from build123d import *

# Parameters (mm, degrees)
F0_R      = 12.7
F1_DEPTH  = 30.1625
F2_W      = 56.912827603
F2_H      = 22.3266
F3_DEPTH  = 44.705
F4_R      = 3.302
F5_R      = 3.302
F6_R      = 6.35
F7_DEPTH  = 22.353
F9_DEPTH  = 19.05
F11_DEPTH = 19.05
F12_R     = 7.874
F13_R     = 5.08


with BuildPart() as f1:
    # F0 (on Front) → F1 (new body, symmetric)
    with BuildSketch(Plane.XZ):
        with BuildLine():
            ThreePointArc((22.352, 22.352), (-15.8052507731, 38.1572507731), (0, 0))
            Line((0, 0), (194.2084, 0))
            Line((194.2084, 0), (194.2084, 22.352))
            Line((194.2084, 22.352), (22.352, 22.352))
        make_face()
        with Locations((0, 22.352)):
            Circle(F0_R, mode=Mode.SUBTRACT)
    extrude(amount=F1_DEPTH, both=True)

    # F2 (on Top) → F3 (cut, through all)
    with BuildSketch(Plane.XY):
        Rectangle(F2_W, F2_H)
    extrude(amount=F3_DEPTH, mode=Mode.SUBTRACT)

    # F4
    f4_edges = [f1.edges().sort_by_distance(p)[0] for p in [
        (22.352, 20.6629, 22.352),
    ]]
    fillet(f4_edges, radius=F4_R)

    # F5
    f5_edges = [f1.edges().sort_by_distance(p)[0] for p in [
        (22.352, -20.6629, 22.352),
    ]]
    fillet(f5_edges, radius=F5_R)

    # F6 (on face) → F7 (cut, through all)
    with BuildSketch(Plane.XY.offset(22.352)):
        with Locations((155.3464, 15.4305)):
            Circle(F6_R)
    extrude(amount=-F7_DEPTH, mode=Mode.SUBTRACT)

    # F8 (on face) → F9 (cut)
    with BuildSketch(Plane.XZ.offset(30.1625)):
        Polygon((117.2464, 0), (117.2464, 22.352), (85.852, 22.352), (91.8464, 0), align=None)
    extrude(amount=-F9_DEPTH, mode=Mode.SUBTRACT)

    # F10 (on face) → F11 (join)
    with BuildSketch(Plane.XZ.offset(30.1625)):
        with BuildLine():
            ThreePointArc((130.1968694519, 57.15), (127.0147572456, 38.5254271914), (117.2464, 22.352))
            Line((117.2464, 22.352), (150.0886, 22.352))
            Line((150.0886, 22.352), (153.3906, 22.352))
            ThreePointArc((153.3906, 22.352), (151.0557334085, 23.3191334085), (150.0886, 25.654))
            Line((150.0886, 25.654), (150.0886, 57.15))
            Line((150.0886, 57.15), (130.1968694519, 57.15))
        make_face()
    extrude(amount=-F11_DEPTH)

    # F12
    f12_edges = [f1.edges().sort_by_distance(p)[0] for p in [
        (194.2084, 0, 22.352),
    ]]
    fillet(f12_edges, radius=F12_R)

    # F13
    f13_edges = [f1.edges().sort_by_distance(p)[0] for p in [
        (150.0886, -20.6375, 57.15),
    ]]
    fillet(f13_edges, radius=F13_R)


solid = f1.part
CAD build for the part. Positions are in the model's coordinates, mm. A direction names the side the tool comes from. Give positions to 0.01 mm unless a question says otherwise; leave off trailing zeros. Loops run counter-clockwise (first coordinate to the right, second up) from the corner with the lowest first, then second, coordinate; pieces in that order, holes last. Notation, with made-up numbers: M 29,15.5 L 47,15.5 A6 ccw 47,25.5 Z; hole C 80,23 d3. An arc over 180 degrees is marked long. Write each question's results on one line, items separated by ' | '.
Q1. Flat gauge pins, fed straight in: P1, Ø4, axis at x = 89, z = 19, coming from the -Y side; P2, Ø15, axis at y = -22, z = 38, coming from the +X side; P3, Ø15, axis at x = 0, z = 22.352, coming from the +Y side; P4, Ø5.5, axis at y = -21.5, z = 9.5, coming from the -X side. Where does each tip first touch, or does it go through?
Geometry check:
P1: stops at y = -11.11 | P2: stops at x = 150.09 | P3: passes through | P4: stops at x = -19.94
Q2. Band-saw the part on D-D on x = 101. Write the cut outline in (y, z), and give its area (3 significant figures).
Geometry check:
outline: M -11.11,0 L 30.16,0 L 30.16,22.35 L -11.11,22.35 Z | area: 923 mm²
Q3. Band-saw the part on B-B on x = -6. Write the cut outline in (y, z), and give its area (3 significant figures).
Geometry check:
outline: M -30.16,0.82 L -11.16,0.82 L -11.16,11.16 L -30.16,11.16 Z; M -30.16,33.55 L -11.16,33.55 L -11.16,43.88 L -30.16,43.88 Z; M 11.16,0.82 L 30.16,0.82 L 30.16,11.16 L 11.16,11.16 Z; M 11.16,33.55 L 30.16,33.55 L 30.16,43.88 L 11.16,43.88 Z | area: 786 mm²
Q4. Band-saw the part on C-C on y = 0. Write the cut outline in (x, z), and give its area (3 significant figures).
Geometry check:
outline: M 28.46,0 L 194.21,0 L 194.21,14.48 A7.87 ccw 186.33,22.35 L 28.46,22.35 Z | area: 3,690 mm²
Q5. Which spindle directions (+Z, -Z, +X, -X, +Y, -Y) get a long thin tool onto all of the face, cutting with end or side? Do faces 5 (the face through (107, 0, 22.352)), 6 (the face through (88.807, -20.771, 11.332)), 7 (the face through (150.089, -21, 39)), 8 (the face through (139, -11.112, 40)). Say none if no direction does.
Geometry check:
face 5: +Z, +Y | face 6: +Z, -Y | face 7: +Z, +X, +Y, -Y | face 8: +Z, +X, -X, +Y
Q6. Band-saw the part on A-A on z = 28.5. Write the cut outline in (x, y).
Geometry check:
outline: M -21.49,-30.16 L -11.11,-30.16 L -11.11,-11.16 L -21.49,-11.16 Z; M -21.49,11.16 L -11.11,11.16 L -11.11,30.16 L -21.49,30.16 Z; M 11.11,-30.16 L 21.49,-30.16 L 21.49,-11.16 L 11.11,-11.16 Z; M 11.11,11.16 L 21.49,11.16 L 21.49,30.16 L 11.11,30.16 Z; M 121.96,-30.16 L 150.09,-30.16 L 150.09,-11.11 L 121.96,-11.11 Z
Q7. Mould opens along X. For faces 1 (the face through (127.11, -20.77, 38.78)), 2 (the face through (148.64, -20.5, 55.62)), 3 (the face through (-16.31, 20.53, 37.636)), 4 (the face through (34, -30.162, 18)) say: pulls with the +X half, pulls with the -X half, needs draft (parallel to the pull), parting line crosses it, or undercut.
Geometry check:
face 1: undercut | face 2: pulls with the +X half | face 3: parting line crosses it | face 4: needs draft
Q8. Probe probe 1 along Y at (x, z) = (28, 20); probe 2 along Z at (x, y) = (0, 24.5); probe 3 along X at (y, z) = (-13.5, 31). List the from-to ranges inside material, lowest first.
Geometry check:
probe 1: y = -30.16 to -11.16, 11.16 to 30.16 | probe 2: z = 0 to 9.65, 35.05 to 44.7 | probe 3: x = -20.61 to -9.3, 9.3 to 20.61, 123.49 to 150.09
